from build123d import *

# Parameters (mm, degrees)
EXTRUSION1_DEPTH = 188.5
ESQUISSE2_R      = 1.5
EXTRUSION2_DEPTH = 267
ESQUISSE3_R      = 1.5
ESQUISSE3_R_2    = 1.723102606
EXTRUSION3_DEPTH = 10


with BuildPart() as part:
    # Esquisse1 → Extrusion1 (new body)
    with BuildSketch(Plane.XY):
        Polygon((-19.477054801, -9.635894737), (-19.477054801, -24.635894737), (-17.977054801, -24.635894737), (-17.977054801, -11.135894737), (-4.477054801, -11.135894737), (-4.477054801, -9.635894737), align=None)
    extrude(amount=EXTRUSION1_DEPTH)

    # Esquisse2 → Extrusion2 (cut)
    with BuildSketch(Plane(origin=(0, -9.635894737, 0), x_dir=(-1, 0, 0), z_dir=(0, 1, 0))):
        with Locations((10.477054801, 8.5)):
            Circle(ESQUISSE2_R)
        with Locations((10.477054801, 181)):
            Circle(ESQUISSE2_R)
        with Locations((10.477054801, 140)):
            Circle(ESQUISSE2_R)
        with Locations((10.477054801, 40)):
            Circle(ESQUISSE2_R)
    extrude(amount=-EXTRUSION2_DEPTH, mode=Mode.SUBTRACT)

    # Esquisse3 → Extrusion3 (cut)
    with BuildSketch(Plane(origin=(-17.977054801, 0, 0), x_dir=(0, 0, -1), z_dir=(1, 0, 0))):
        with Locations((-40, -20.135894737)):
            Circle(ESQUISSE3_R)
        with Locations((-140, -20.135894737)):
            Circle(ESQUISSE3_R)
        with Locations((-181, -20.135894737)):
            Circle(ESQUISSE3_R)
        with Locations((-7.5, -17.135894737)):
            Circle(ESQUISSE3_R_2)
    extrude(amount=-EXTRUSION3_DEPTH, mode=Mode.SUBTRACT)


solid = part.part
Here's how the part is built. I have some questions about the finished solid (model axes, mm). A direction names the side the tool comes from. Coordinates: 2 decimals unless noted, no trailing zeros. Order: outer loops, then holes, each group sorted by start corner. A loop starts at its lowest first (then second) coordinate and runs counter-clockwise, first axis right, second up. Notation, with made-up numbers: M 21.25,29.5 L 62.25,29.5 A14 ccw 62.25,55.5 Z; hole C -40,29.25 d3. An arc over 180 degrees is marked long. Answer as CSV lines item,"result". Start each with the question number.
1. I want a section at B-B, the plane x = -6.5. Write out the boundary of the cut face in (y, z).
2. On a 3-axis mill with a long thin cutter (end or side, diameter ignored), from which of +Z, -Z, +X, -X, +Y, -Y can I reach the whole of each face in a straight line? I mean faces 4 (the cylindrical face through (-10.282, -10.375, 182.487)), 5 (the flat face through (-11, -11.136, 93)). Say none if no direction works.
3. We'd pull the mould along X, two halves only. Please class faces 1 (the cylindrical face through (-18.7, -20.1, 141.5)), 2 (the cylindrical face through (-10.152, -10.375, 38.536)), 3 (the flat face through (-19.477, -17, 93)): released by +X, released by -X, zero draft, split by the parting line, or undercut.
4. For pin 1 (3 mm diameter, centred on x = -10.5, z = 164, fed in from -Y); pin 2 (2 mm diameter, centred on y = -16.5, z = 71.5, fed in from +X), each with a flat end and sliding along its axis, tell me the tip position at first contact or that it passes through.
5. I want a section at A-A, the plane z = 155.5. Write out the boundary of the cut face in (x, y), and give its area (4 significant figures).
6. I need wall thicknesses on line 1 (X direction, y = -20, z = 53); line 2 (Y direction, x = -4.75, z = 126). Which ranges of each line are inside material? Lowest first, please. Write a range as [from, to].
Recorded:
1,outline,"M -11.14,0 L -9.64,0 L -9.64,188.5 L -11.14,188.5 Z"
2,face 4,"+Y, -Y"
2,face 5,"+Z, -Z, +X, -Y"
3,face 1,"zero draft"
3,face 2,"undercut"
3,face 3,"released by -X"
4,pin 1,"stops at y = -11.14"
4,pin 2,"stops at x = -17.98"
5,outline,"M -19.48,-24.64 L -17.98,-24.64 L -17.98,-11.14 L -4.48,-11.14 L -4.48,-9.64 L -19.48,-9.64 Z"
5,area,"42.75 mm2"
6,line 1,"x = [-19.48, -17.98]"
6,line 2,"y = [-11.14, -9.64]"
